Verification items for this drawing (mm, ordinates from the low corner). A direction names the side the tool comes from. Give positions to 0.01 mm unless a question says otherwise; leave off trailing zeros. Write each loop counter-clockwise with the first axis right and the second up, starting at its lowest first coordinate (ties: lowest second). Pieces come first, ordered by that corner, then holes. Notation, with made-up numbers: (40, 87.25) -> (46, 87.25) arc R26 ccw to (46, 116.25) -> close; hole circle Ø7 at (8, 63). An arc over 180 degrees is marked (long way). One line per item, written item: value.
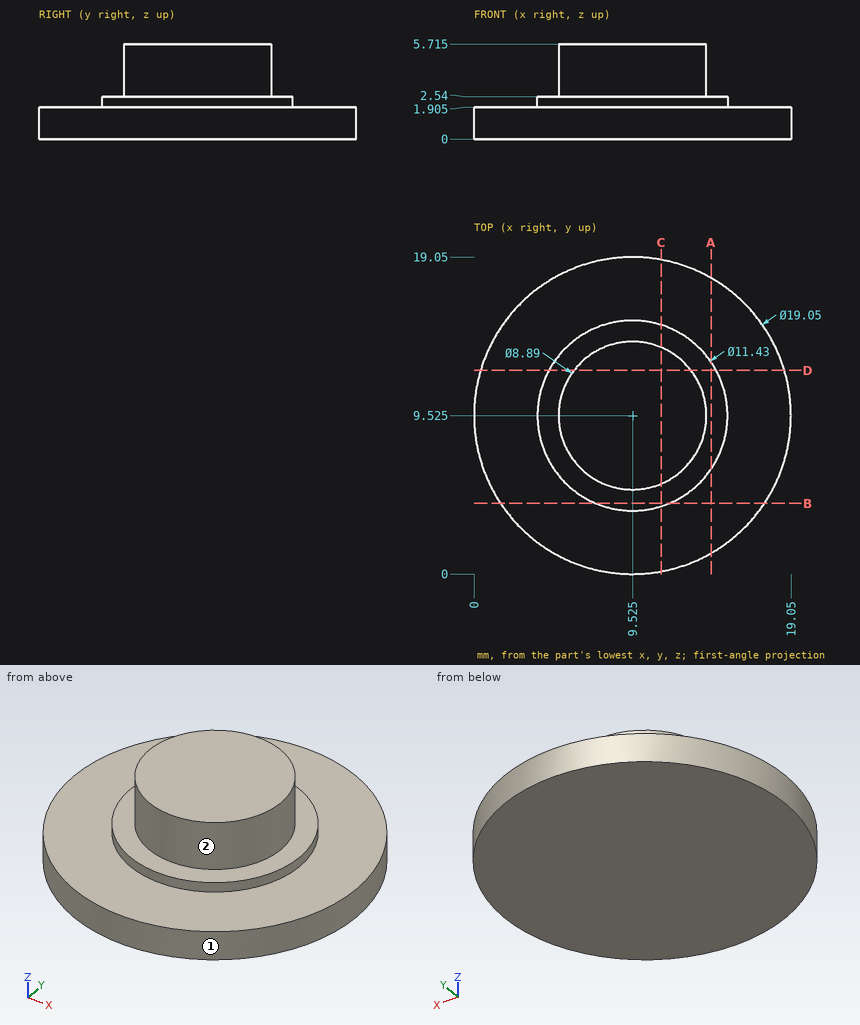
1) Sectioned sample at A-A on x = 14.25. Record the cut outline in (y, z) (3 decimals), plus the area to 3 significant figures.
Verdict:
outline: (1.255, 0) -> (17.795, 0) -> (17.795, 1.905) -> (12.74, 1.905) -> (12.74, 2.54) -> (6.31, 2.54) -> (6.31, 1.905) -> (1.255, 1.905) -> close
area: 35.6 mm^2
2) Sectioned sample at B-B on y = 4.25. Record the cut outline in (x, z) (3 decimals).
Verdict:
outline: (1.594, 0) -> (17.456, 0) -> (17.456, 1.905) -> (11.724, 1.905) -> (11.724, 2.54) -> (7.326, 2.54) -> (7.326, 1.905) -> (1.594, 1.905) -> close
3) Tool access check on the marked faces 1 and 2. Record the directions out of +Z, -Z, +X, -X, +Y, -Y that give a thin tool (end or side, any length) a straight path to the whole face; none if there is none.
Verdict:
face 1: +Z, -Z
face 2: +Z
4) Scan lines: probe 1 along Z at (x, y) = (16, 12.25) (3 decimals); probe 2 along Z at (x, y) = (7.75, 14); probe 3 along X at (y, z) = (8.75, 0.8). Record each from-to range of solid material in increasing order.
Verdict:
probe 1: 0 to 1.905
probe 2: 0 to 2.54
probe 3: 0.03 to 19.02
5) Depth check by flat-ended pin: pin 1 Ø2 at (x, y) = (14, 12) entering from +Z (3 decimals); pin 2 Ø2 at (y, z) = (7, 3) entering from -X; pin 3 Ø1 at (y, z) = (10.5, 4) entering from +X; pin 4 Ø2 at (x, z) = (3, 5) entering from +Y. Enter the tip coordinate at first touch or a pass-through.
Verdict:
pin 1: z = 5.715
pin 2: x = 4.05
pin 3: x = 13.94
pin 4: through
6) Sectioned sample at D-D on y = 12.25. Record the cut outline in (x, z) (1 decimal).
Verdict:
outline: (0.4, 0) -> (18.7, 0) -> (18.7, 1.9) -> (14.5, 1.9) -> (14.5, 2.5) -> (13, 2.5) -> (13, 5.7) -> (6, 5.7) -> (6, 2.5) -> (4.5, 2.5) -> (4.5, 1.9) -> (0.4, 1.9) -> close
7) Sectioned sample at C-C on x = 11.25. Record the cut outline in (y, z) (1 decimal), plus the area to 3 significant figures.
Verdict:
outline: (0.2, 0) -> (18.9, 0) -> (18.9, 1.9) -> (15, 1.9) -> (15, 2.5) -> (13.6, 2.5) -> (13.6, 5.7) -> (5.4, 5.7) -> (5.4, 2.5) -> (4.1, 2.5) -> (4.1, 1.9) -> (0.2, 1.9) -> close
area: 68.6 mm^2
